```python
from build123d import *

# Parameters (mm, degrees)
BOSS_EXTRUDE1_DEPTH = 41
CUT_EXTRUDE1_DEPTH  = 11
BOSS_EXTRUDE4_DEPTH = 2
FILLET1_R           = 1


with BuildPart() as part:
    # Sketch2 → Boss-Extrude1 (new, symmetric)
    with BuildSketch(Plane(origin=(0, 0, 0), x_dir=(0, 0, -1), z_dir=(1, 0, 0))):
        with BuildLine():
            Line((-0.141756815, 2.245530005), (-1.922649731, 5.330127019))
            Line((-1.922649731, 5.330127019), (-59, 5.330127019))
            Line((-59, 5.330127019), (-59, 3.330127019))
            Line((-59, 3.330127019), (-3.077350269, 3.330127019))
            Line((-3.077350269, 3.330127019), (-1.873807622, 1.245530005))
            ThreePointArc((-1.873807622, 1.245530005), (-1.983045954, -1.063028101), (0, -2.25))
            Line((0, -2.25), (0, -1.25))
            ThreePointArc((0, -1.25), (-0.883883476, 0.883883476), (1.25, 0))
            Line((1.25, 0), (2.25, 0))
            ThreePointArc((2.25, 0), (1.540056357, 1.640343384), (-0.141756815, 2.245530005))
        make_face()
    extrude(amount=BOSS_EXTRUDE1_DEPTH, both=True)

    # Sketch4 → Cut-Extrude1 (cut)
    with BuildSketch(Plane(origin=(41, 0, 0), x_dir=(0, 0, -1), z_dir=(1, 0, 0))):
        with BuildLine():
            Line((-3.077350269, 3.330127019), (-1.873807622, 1.245530005))
            ThreePointArc((-1.873807622, 1.245530005), (-1.983045954, -1.063028101), (0, -2.25))
            Line((0, -2.25), (0, -1.25))
            ThreePointArc((0, -1.25), (-0.883883476, 0.883883476), (1.25, 0))
            Line((1.25, 0), (2.25, 0))
            ThreePointArc((2.25, 0), (1.540056357, 1.640343384), (-0.141756815, 2.245530005))
            Line((-0.141756815, 2.245530005), (-1.922649731, 5.330127019))
            Line((-1.922649731, 5.330127019), (-5.922649731, 5.330127019))
            Line((-5.922649731, 5.330127019), (-5.922649731, 3.330127019))
            Line((-5.922649731, 3.330127019), (-3.077350269, 3.330127019))
        make_face()
    cut_extrude1 = extrude(amount=-CUT_EXTRUDE1_DEPTH, mode=Mode.SUBTRACT)

    # Mirror1: Cut-Extrude1 across plane
    add(cut_extrude1.mirror(Plane(origin=(0, 0, 0), x_dir=(0, 0, 1), z_dir=(1, 0, 0))), mode=Mode.SUBTRACT)

    # Sketch8 → Boss-Extrude4 (add)
    with BuildSketch(Plane(origin=(0, 5.330127019, 0), x_dir=(1, 0, 0), z_dir=(0, 1, 0))):
        with BuildLine():
            Line((0, -59), (-9.997341071, -59))
            ThreePointArc((-9.997341071, -59), (0, -64.816412092), (9.997341071, -59))
            Line((9.997341071, -59), (0, -59))
        make_face()
    extrude(amount=-BOSS_EXTRUDE4_DEPTH)

    # Fillet1
    fillet1_edges = [part.edges().sort_by_distance(p)[0] for p in [
        (-35.5, 5.330127019, 5.922649731),
        (35.5, 5.330127019, 5.922649731),
        (-41, 4.330127019, 59),
        (41, 4.330127019, 59),
        (41, 5.330127019, 32.461324865),
        (-25.498670535, 5.330127019, 59),
        (25.498670535, 5.330127019, 59),
        (-41, 5.330127019, 32.461324865),
        (41, 4.330127019, 5.922649731),
        (-41, 4.330127019, 5.922649731),
        (30, 5.330127019, 3.922649731),
        (-30, 5.330127019, 3.922649731),
        (0, 5.330127019, 1.922649731),
        (0, 3.330127019, 64.816412092),
        (0, -1.25, 0),
        (0, 0, -1.25),
    ]]
    fillet(fillet1_edges, radius=FILLET1_R - 0.0001)  # a hair under: the kernel refuses the full size


solid = part.part
```
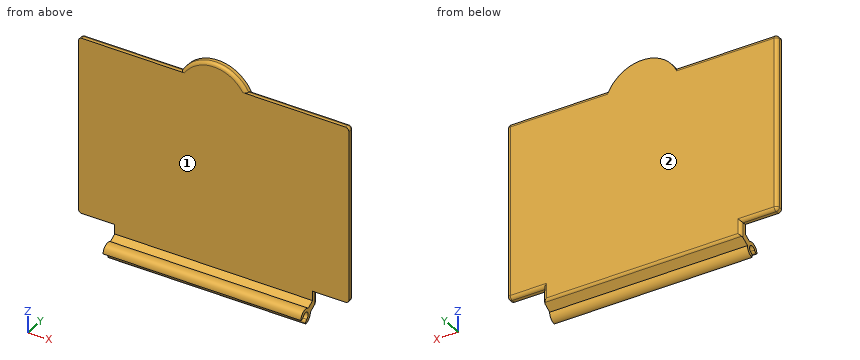
Geometry check sheet. Reference: the model listing, model coordinates, mm. Face numbers are marked on the shaded views. A direction names the side the tool comes from. Round coordinates to 2 decimals unless told otherwise and drop trailing zeros. Loops run counter-clockwise (first coordinate to the right, second up) from the corner with the lowest first, then second, coordinate; pieces in that order, holes last. Notation, with made-up numbers: M 9,60.5 L 54,60.5 A7 cw 54,70.5 Z; hole C -30,26 d8. An arc over 180 degrees is marked long. Return JSON: item names as keys, results as strings. Group by question number.
(1) Section check C-C, the plane x = 33.5. Enter the section's corners in (y, z), and give its area (3 significant figures).
(2) Scan lines: line 1 along Y through (x, z) = (26, 36); line 2 along X through (y, z) = (4.5, 22.5); line 3 along Z through (x, y) = (-10, -0.25). Record each from-to range of solid material in increasing order. Write a range as [from, to].
(3) Section check B-B, the plane z = 10.5. Enter the section's corners in (x, y).
(4) Section check A-A, the plane x = 18.5. Enter the section's corners in (y, z).
(5) Set-up check for the marked faces 1 and 2: record each of +Z, -Z, +X, -X, +Y, -Y from which the full face is reachable in a straight line by a thin tool's end or side.
(6) Go/stop test with flat-tipped pins: pin 1 (3 mm diameter, centred on y = 0, z = 0, fed in from -X); pin 2 (3.5 mm diameter, centred on y = -0.5, z = 1, fed in from +X); pin 3 (0.5 mm diameter, centred on x = -26.5, y = 4, fed in from +Z); pin 4 (1.5 mm diameter, centred on x = 31.5, y = 1.5, fed in from -Z). Record where each tip stops, or that it passes through.
Data:
{
 "1": {"outline": "M 3.33,5.92 L 4.33,5.92 A1 ccw 5.33,6.92 L 5.33,58 A1 ccw 4.33,59 L 3.33,59 Z", "area": "106 mm²"},
 "2": {"line 1": "[3.33, 5.33]", "line 2": "[-40.99, 40.99]", "line 3": "[1.22, 2.24]"},
 "3": {"outline": "M -41,3.33 L 41,3.33 L 41,4.33 A1 ccw 40,5.33 L -40,5.33 A1 ccw -41,4.33 Z"},
 "4": {"outline": "M -2.25,0 L -2.02,0 A1 ccw -1.12,0.56 A1.25 cw long 0.56,-1.12 A1 ccw 0,-2.02 L 0,-2.25 A2.25 ccw 2.25,0.14 L 4.83,1.63 A1 ccw 5.33,2.5 L 5.33,58 A1 ccw 4.33,59 L 3.33,59 L 3.33,3.08 L 1.25,1.87 A2.25 ccw Z"},
 "5": {"face 1": "+Z, +X, -X, -Y", "face 2": "+Z, -Z, +X, -X, +Y"},
 "6": {"pin 1": "x = -30", "pin 2": "x = 30", "pin 3": "z = 59", "pin 4": "through"}
}
